```python
from build123d import *
from build123d.topology import SkipClean

# Parameters (mm, degrees)
SKETCH1_R           = 9.5
SKETCH1_W           = 2
SKETCH1_H           = 18.894444
BOSS_EXTRUDE1_DEPTH = 5
SKETCH1_3_W         = 2
SKETCH1_3_H         = 2
BOSS_EXTRUDE2_DEPTH = 22
CUT_EXTRUDE2_REACH  = 32.778
CUT_EXTRUDE2_START  = 5
SKETCH1_4_W         = 2
SKETCH1_4_H         = 18.894444
SKETCH1_4_W_2       = 18.894444
SKETCH1_4_H_2       = 2
CHAMFER1_SIZE       = 0.5
SKETCH7_R           = 3
CUT_EXTRUDE3_DEPTH  = 20


with BuildPart() as part:
    # Sketch1 → Boss-Extrude1 (new body)
    with BuildSketch(Plane.XY):
        Circle(SKETCH1_R)
        Rectangle(SKETCH1_W, SKETCH1_H)
    extrude(amount=BOSS_EXTRUDE1_DEPTH)

    # Sketch1_3 → Boss-Extrude2 (add)
    with BuildSketch(Plane.XY):
        with BuildLine():
            Line((-5.408327, 1), (-1, 1))
            Line((-1, 1), (-1, 5.408327))
            ThreePointArc((-1, 5.408327), (-3.889087, 3.889087), (-5.408327, 1))
        make_face()
        with BuildLine():
            ThreePointArc((-5.408327, -1), (-3.889087, -3.889087), (-1, -5.408327))
            Line((-1, -5.408327), (-1, -1))
            Line((-1, -1), (-5.408327, -1))
        make_face()
        with BuildLine():
            Line((-5.408327, -1), (-1, -1))
            Line((-1, -1), (-1, 1))
            Line((-1, 1), (-5.408327, 1))
            ThreePointArc((-5.408327, 1), (-5.5, 0), (-5.408327, -1))
        make_face()
        with BuildLine():
            Line((1, 5.408327), (1, 1))
            Line((1, 1), (5.408327, 1))
            ThreePointArc((5.408327, 1), (3.889087, 3.889087), (1, 5.408327))
        make_face()
        with BuildLine():
            Line((1, -1), (1, -5.408327))
            ThreePointArc((1, -5.408327), (3.889087, -3.889087), (5.408327, -1))
            Line((5.408327, -1), (1, -1))
        make_face()
        with BuildLine():
            Line((1, 1), (1, -1))
            Line((1, -1), (5.408327, -1))
            ThreePointArc((5.408327, -1), (5.477034, -0.502097), (5.5, 0))
            ThreePointArc((5.5, 0), (5.477034, 0.502097), (5.408327, 1))
            Line((5.408327, 1), (1, 1))
        make_face()
        with BuildLine():
            Line((-1, 5.408327), (-1, 1))
            Line((-1, 1), (1, 1))
            Line((1, 1), (1, 5.408327))
            ThreePointArc((1, 5.408327), (0, 5.5), (-1, 5.408327))
        make_face()
        with BuildLine():
            Line((-1, -1), (-1, -5.408327))
            ThreePointArc((-1, -5.408327), (0, -5.5), (1, -5.408327))
            Line((1, -5.408327), (1, -1))
            Line((1, -1), (-1, -1))
        make_face()
        Rectangle(SKETCH1_3_W, SKETCH1_3_H)
    extrude(amount=-BOSS_EXTRUDE2_DEPTH)

    # Sketch2 → Revolve1 (revolve)
    with BuildSketch(Plane(origin=(0, 0, 0), x_dir=(0, 0, -1), z_dir=(1, 0, 0)), mode=Mode.PRIVATE) as revolve1_sk:
        with BuildLine():
            Line((-5, 9.5), (-5, 0))
            Line((-5, 0), (-7.5, 0))
            ThreePointArc((-7.5, 0), (-6.864539, 4.911721), (-5, 9.5))
        make_face()
    revolve(revolve1_sk.sketch.rotate(Axis((0, 0, 0), (0, 0, 1)), 270), axis=Axis((0, 0, 0), (0, 0, 1)))

    # Sketch1_4 → Cut-Extrude2 (cut, up to next)
    with BuildSketch(Plane.XY.offset(CUT_EXTRUDE2_START), mode=Mode.PRIVATE) as cut_extrude2_sk1:
        Rectangle(SKETCH1_4_W, SKETCH1_4_H)
    cut_extrude2_tool1 = extrude(cut_extrude2_sk1.sketch, amount=CUT_EXTRUDE2_REACH, mode=Mode.PRIVATE) & part.part
    # Sketch1_4 → Cut-Extrude2 (cut, up to next)
    with BuildSketch(Plane.XY.offset(CUT_EXTRUDE2_START), mode=Mode.PRIVATE) as cut_extrude2_sk2:
        Rectangle(SKETCH1_4_W_2, SKETCH1_4_H_2)
    cut_extrude2_tool2 = extrude(cut_extrude2_sk2.sketch, amount=CUT_EXTRUDE2_REACH, mode=Mode.PRIVATE) & part.part
    add(cut_extrude2_tool1.solids().sort_by_distance((0, 0, 5))[0], mode=Mode.SUBTRACT)
    add(cut_extrude2_tool2.solids().sort_by_distance((0, 0, 5))[0], mode=Mode.SUBTRACT)

    # Chamfer1
    chamfer1_edges = [part.edges().sort_by_distance(p)[0] for p in [
        (-9.5, 0, 0),
    ]]
    chamfer(chamfer1_edges, length=CHAMFER1_SIZE)

    # Sketch7 → Cut-Extrude3 (cut)
    with SkipClean():  # the faces are left unmerged after this step: merging them gives an invalid solid
        with BuildSketch(Plane(origin=(0, 0, -22), x_dir=(-1, 0, 0), z_dir=(0, 0, -1))):
            Circle(SKETCH7_R)
        extrude(amount=-CUT_EXTRUDE3_DEPTH, mode=Mode.SUBTRACT)


solid = part.part
```
Model file for the job. Use its own axes, mm. A direction names the side the tool comes from. Round coordinates to 2 decimals unless told otherwise and drop trailing zeros. Loops run counter-clockwise (first coordinate to the right, second up) from the corner with the lowest first, then second, coordinate; pieces in that order, holes last. Notation, with made-up numbers: M -6.75,-27 L 29.25,-27 A25 cw 29.25,0 Z; hole C -34.5,8 d10. An arc over 180 degrees is marked long. Put each result on its own line as item: value. Start each with the question number.
Item 1: Drop flat-ended pins along their axis: P1, Ø10, axis at x = 6.5, y = 6.5, coming from the +Z side; P2, Ø8, axis at y = -6.5, z = -10.5, coming from the +X side; P3, Ø3.5, axis at x = 0, y = 0, coming from the +Z side; P4, Ø1.5, axis at x = 2.5, z = -2.5, coming from the -Y side. Give the stop position or say it passes through.
Item 2: Drill centre lines: line 1 along Y through (x, z) = (0, -7.5); line 2 along X through (y, z) = (2.5, -18.5); line 3 along X through (y, z) = (2, -13.25). Where is each one in solid material? Low to high.
Item 3: Cut at A-A (z = 2.5). List the corners of the cut face in (x, y), then the cut area to 3 significant figures.
Item 4: 3-axis set-ups, long thin cutter, end or side, ignore diameter. For faces 5 (the face through (1, 4, 6)), 6 (the face through (2.4, -2.4, -22)), 7 (the face through (4, 1, 6)), 8 (the face through (0, 0, -2)): which of +Z, -Z, +X, -X, +Y, -Y reach the whole face in a straight line?
Item 5: Mould opens along X. For faces 1 (the face through (1, -4, 6)), 2 (the face through (4.38, -8.43, 2.72)), 3 (the face through (-4, -4, 0)), 4 (the face through (3, 0, -12)) say: released by +X, released by -X, zero draft, split by the parting line, or undercut.
Answer block:
1. P1: z = 7.04
1. P2: x = 4.9
1. P3: z = 7.45
1. P4: y = -5.21
2. line 1: -5.5 to -3, 3 to 5.5
2. line 2: -4.9 to -1.66, 1.66 to 4.9
2. line 3: -5.12 to -2.24, 2.24 to 5.12
3. outline: C 0,0 d19
3. area: 284 mm2
4. face 5: +Z, +Y, -Y
4. face 6: -Z, +X, -X, +Y, -Y
4. face 7: +Z, +X, -X
4. face 8: -Z
5. face 1: undercut
5. face 2: split by the parting line
5. face 3: zero draft
5. face 4: undercut
